Autodesk Fusion 360 part; units mm, degrees
sketch "Sketch1" plane through (0, 0, 0) normal (0, 0, 1) x (1, 0, 0)
  line L0 (10, 20.25) -> (-10, 20.25)
  line L1 (-10, 20.25) -> (-10, -20.25)
  line L2 (-10, -20.25) -> (10, -20.25)
  line L3 (10, -20.25) -> (10, 20.25)
  line L4 (10, 20.25) -> (-10, -20.25) construction
  line L5 (-10, 20.25) -> (10, -20.25) construction
  dimension "d1" = 20
  dimension "d2" = 40.5
extrude "Extrude1" add sketch "Sketch1" along normal blind 21.5
sketch "Sketch2" plane through (0, 0, 21.5) normal (0, 0, 1) x (-1, 0, 0)
  line L0 (-10, 20.25) -> (-10, -20.25)
  line L1 (-10, -20.25) -> (10, -20.25)
  line L2 (10, -20.25) -> (10, 20.25)
  line L3 (10, 20.25) -> (-10, 20.25)
  line L4 (-8, -18.25) -> (8, -18.25)
  line L5 (8, -18.25) -> (8, 18.25)
  line L6 (8, 18.25) -> (-8, 18.25)
  line L7 (-8, 18.25) -> (-8, -18.25)
  line L8 (-8, -18.25) -> (8, 18.25) construction
  line L9 (8, -18.25) -> (-8, 18.25) construction
  line L10 (-9, -19.25) -> (9, -19.25)
  line L11 (9, -19.25) -> (9, 19.25)
  line L12 (9, 19.25) -> (-9, 19.25)
  line L13 (-9, 19.25) -> (-9, -19.25)
  line L14 (-9, -19.25) -> (9, 19.25) construction
  line L15 (9, -19.25) -> (-9, 19.25) construction
  dimension "d5" = 1
  dimension "d6" = 1
  dimension "d7" = 1
  dimension "d8" = 1
extrude "Extrude2" add sketch "Sketch2" along normal blind 1 contours L10 L11 L12 L13
sketch "Sketch3" plane through (0, 0, 21.5) normal (0, 0, 1) x (-1, 0, 0)
  line L0 (-8, -18.25) -> (8, -18.25)
  line L1 (8, -18.25) -> (8, 18.25)
  line L2 (8, 18.25) -> (-8, 18.25)
  line L3 (-8, 18.25) -> (-8, -18.25)
  circle A0 centre (0, 10.25) radius 2
  line L4 (10, 20.25) -> (-10, 20.25)
  circle A1 centre (0, -0.75) radius 0.75
  circle A2 centre (0, -10.25) radius 3
  line L5 (-10, -20.25) -> (10, -20.25)
  circle A3 centre (0, -10.25) radius 4
  circle A4 centre (0, 10.25) radius 4
  dimension "d11" = 4
  dimension "d12" = 10
  dimension "d13" = 11
  dimension "d14" = 9.5
  dimension "d16" = 10
  dimension "d17" = 1.5
  dimension "d18" = 6
  dimension "d19" = 8
  dimension "d20" = 8
extrude "Extrude3" add sketch "Sketch3" along normal blind 5 contours A3
extrude "Extrude4" add sketch "Sketch3" along normal blind 5 contours A4
sketch "Sketch4" plane through (0, 0, 26.5) normal (0, 0, 1) x (-1, 0, 0)
  circle A0 centre (0, 10.25) radius 2
  circle A1 centre (0, 10.25) radius 4
  circle A2 centre (0, 10.25) radius 3
  dimension "d25" = 6
extrude "Extrude5" cut sketch "Sketch4" against normal blind 2.5 contours A1
extrude "Extrude6" cut sketch "Sketch3" against normal blind 1.5 contours A1
sketch "Sketch5" plane through (0, 0, 0) normal (0, 0, -1) x (1, 0, 0)
  line L0 (10, -20.25) -> (10, 20.25)
  line L1 (10, 20.25) -> (-10, 20.25)
  line L2 (-10, 20.25) -> (-10, -20.25)
  line L3 (-10, -20.25) -> (10, -20.25)
  line L4 (7.5, 18) -> (-7.5, 18) construction
  line L5 (-7.5, 18) -> (-7.5, -18) construction
  line L6 (-7.5, -18) -> (7.5, -18) construction
  line L7 (7.5, -18) -> (7.5, 18) construction
  line L8 (7.5, 18) -> (-7.5, -18) construction
  line L9 (-7.5, 18) -> (7.5, -18) construction
  circle A0 centre (-7.5, 18) radius 0.875
  circle A1 centre (7.5, 18) radius 0.875
  circle A2 centre (7.5, -18) radius 0.875
  circle A3 centre (-7.5, -18) radius 0.875
  dimension "d30" = 15
  dimension "d31" = 36
  dimension "d32" = 1.75
extrude "Extrude7" cut sketch "Sketch5" against normal blind 27 contours A0 | A1 | A2 | A3
sketch "Sketch6" plane through (0, 0, 0) normal (0, 0, -1) x (1, 0, 0)
  circle A0 centre (7.5, 18) radius 0.875
  circle A1 centre (7.5, -18) radius 0.875
  circle A2 centre (-7.5, 18) radius 0.875
  circle A3 centre (-7.5, -18) radius 0.875
  line L0 (10, -20.25) -> (10, 20.25)
  line L1 (10, 20.25) -> (-10, 20.25)
  line L2 (-10, 20.25) -> (-10, -20.25)
  line L3 (-10, -20.25) -> (10, -20.25)
  circle A4 centre (-7.5, 18) radius 1.875
  circle A5 centre (7.5, 18) radius 1.875
  circle A6 centre (7.5, -18) radius 1.875
  circle A7 centre (-7.5, -18) radius 1.875
  line L4 (9, 19.25) -> (-9, 19.25)
  line L5 (-9, 19.25) -> (-9, -19.25)
  line L6 (-9, -19.25) -> (9, -19.25)
  line L7 (9, -19.25) -> (9, 19.25)
  line L8 (9, 19.25) -> (-9, -19.25) construction
  line L9 (-9, 19.25) -> (9, -19.25) construction
  dimension "d35" = 3.75
  dimension "d36" = 1
  dimension "d37" = 1
extrude "Extrude8" cut sketch "Sketch6" against normal up to surface (19.5 mm away) contours A4 A5 A6 A7 L4 L5 L6 L7
extrude "Extrude9" cut 1 faces at (0.1483, -10.9, 21.5) along direction (0, 0, -1) blind 15
sketch "Sketch8" plane through (0, 0, 26.5) normal (0, 0, 1) x (-1, 0, 0)
  circle A0 centre (0, -10.25) radius 3
  circle A1 centre (0, -10.25) radius 4
  circle A2 centre (0, -10.25) radius 4
extrude "Extrude10" add sketch "Sketch8" against normal blind 2.5 contours A0
ref_plane "WorkPlane1" through (0, 6.25, 22) normal (0, -1, 0) x (1, 0, 0)
sketch "Sketch10" plane through (0, 6.25, 22) normal (0, -1, 0) x (1, 0, 0)
  line L0 (-4, 2) -> (4, 2)
  line L1 (4, 2) -> (4, -0.5)
  line L2 (4, -0.5) -> (-4, -0.5)
  line L3 (-4, -0.5) -> (-4, 2)
extrude "Extrude11" cut sketch "Sketch10" against normal blind 2
sketch "Sketch11" plane through (0, 0, 26.5) normal (0, 0, 1) x (-1, 0, 0)
  circle A0 centre (0, -10.25) radius 4
  circle A1 centre (0, -10.25) radius 0.75
  dimension "d47" = 1.5
extrude "Extrude12" cut sketch "Sketch11" against normal blind 1.5 contours A1
sketch "Sketch12" plane through (0, 0, 21.5) normal (0, 0, 1) x (-1, 0, 0)
  arc A0 (-3.4641, -8.25) -> (3.4641, -8.25) centre (0, -10.25) ccw
  line L0 (-3.4641, -8.25) -> (-2.2361, -8.25)
  arc A1 (-2.2361, -8.25) -> (2.2361, -8.25) centre (0, -10.25) ccw
  line L1 (2.2361, -8.25) -> (3.4641, -8.25)
  arc A2 (-8, 17.2819) -> (-6.6615, 18.25) centre (-7.5, 18) ccw
  line L2 (-8, 17.2819) -> (-8, -17.2819)
  arc A3 (-6.6615, -18.25) -> (-8, -17.2819) centre (-7.5, -18) ccw
  line L3 (-6.6615, -18.25) -> (6.6615, -18.25)
  arc A4 (8, -17.2819) -> (6.6615, -18.25) centre (7.5, -18) ccw
  line L4 (8, -17.2819) -> (8, 17.2819)
  arc A5 (6.6615, 18.25) -> (8, 17.2819) centre (7.5, 18) ccw
  line L5 (6.6615, 18.25) -> (-6.6615, 18.25)
  circle A6 centre (0, -0.75) radius 0.75
  circle A7 centre (0, 10.25) radius 4
  circle A8 centre (0, -10.25) radius 3
  dimension "d50" = 6
extrude "Extrude13" cut sketch "Sketch12" against normal blind 4 contours A1 A8
sketch "Sketch13" plane through (0, 0, 21.5) normal (0, 0, 1) x (-1, 0, 0)
  arc A0 (2.2361, -8.25) -> (-2.2361, -8.25) centre (0, -10.25) ccw
  line L0 (2.2361, -8.25) -> (3.4641, -8.25)
  arc A1 (-3.4641, -8.25) -> (3.4641, -8.25) centre (0, -10.25) ccw
  line L1 (-3.4641, -8.25) -> (-2.2361, -8.25)
  arc A2 (-8, 17.2819) -> (-6.6615, 18.25) centre (-7.5, 18) ccw
  line L2 (-8, 17.2819) -> (-8, -17.2819)
  arc A3 (-6.6615, -18.25) -> (-8, -17.2819) centre (-7.5, -18) ccw
  line L3 (-6.6615, -18.25) -> (6.6615, -18.25)
  arc A4 (8, -17.2819) -> (6.6615, -18.25) centre (7.5, -18) ccw
  line L4 (8, -17.2819) -> (8, 17.2819)
  arc A5 (6.6615, 18.25) -> (8, 17.2819) centre (7.5, 18) ccw
  line L5 (6.6615, 18.25) -> (-6.6615, 18.25)
  circle A6 centre (0, -0.75) radius 0.75
  circle A7 centre (0, 10.25) radius 4
  line L6 (-12.9231, -4.25) -> (12.9231, -4.25)
  line L7 (12.9231, -4.25) -> (12.9231, 2.75)
  line L8 (12.9231, 2.75) -> (-12.9231, 2.75)
  line L9 (-12.9231, 2.75) -> (-12.9231, -4.25)
  line L10 (-12.9231, -4.25) -> (12.9231, 2.75) construction
  line L11 (12.9231, -4.25) -> (-12.9231, 2.75) construction
  point P0 (0, -0.75)
  dimension "d53" = 7
extrude "Extrude14" cut sketch "Sketch13" along normal blind 3 contours L2 L6 L8 L9 | L4 L6 L7 L8
fillet "Fillet1" radius 0.35 8 edges at (-9, 4.25, 22) (-8, 4.25, 22) (-9, -2.75, 22) (-8, -2.75, 22) (8, 4.25, 22) (9, 4.25, 22) (8, -2.75, 22) (9, -2.75, 22)
fillet "Fillet2" radius 1 4 edges at (-10, -20.25, 10.75) (10, -20.25, 10.75) (-10, 20.25, 10.75) (10, 20.25, 10.75)
sketch "Sketch14" plane through (0, 0, 19.5) normal (0, 0, -1) x (1, 0, 0)
  circle A0 centre (0, -10.25) radius 3
  circle A1 centre (0, 10.25) radius 2
  arc A2 (-6.1025, -19.25) -> (-9, -16.875) centre (-7.5, -18) ccw
  line L0 (-6.1025, -19.25) -> (6.1025, -19.25)
  arc A3 (9, -16.875) -> (6.1025, -19.25) centre (7.5, -18) ccw
  line L1 (9, -16.875) -> (9, 16.875)
  arc A4 (6.1025, 19.25) -> (9, 16.875) centre (7.5, 18) ccw
  line L2 (6.1025, 19.25) -> (-6.1025, 19.25)
  arc A5 (-9, 16.875) -> (-6.1025, 19.25) centre (-7.5, 18) ccw
  line L3 (-9, 16.875) -> (-9, -16.875)
  circle A6 centre (0, -10.25) radius 8.5
  circle A7 centre (0, -10.25) radius 9.5
  dimension "d60" = 17
  dimension "d61" = 1
extrude "Extrude15" add sketch "Sketch14" along normal blind 12 contours A2 L0 A3 L1 L3 A7
sketch "Sketch15" plane through (0, 0, 19.5) normal (0, 0, -1) x (1, 0, 0)
  circle A0 centre (0, 10.25) radius 2
  arc A1 (9, -7.2086) -> (-9, -7.2086) centre (0, -10.25) ccw
  line L0 (9, -7.2086) -> (9, 16.875)
  arc A2 (6.1025, 19.25) -> (9, 16.875) centre (7.5, 18) ccw
  line L1 (6.1025, 19.25) -> (-6.1025, 19.25)
  arc A3 (-9, 16.875) -> (-6.1025, 19.25) centre (-7.5, 18) ccw
  line L2 (-9, 16.875) -> (-9, -7.2086)
  line L3 (5, 15.75) -> (-5, 15.75)
  line L4 (-5, 15.75) -> (-5, 4.75)
  line L5 (-5, 4.75) -> (5, 4.75)
  line L6 (5, 4.75) -> (5, 15.75)
  line L7 (5, 15.75) -> (-5, 4.75) construction
  line L8 (-5, 15.75) -> (5, 4.75) construction
  line L9 (6, 16.75) -> (-6, 16.75)
  line L10 (-6, 16.75) -> (-6, 3.75)
  line L11 (-6, 3.75) -> (6, 3.75)
  line L12 (6, 3.75) -> (6, 16.75)
  line L13 (6, 16.75) -> (-6, 3.75) construction
  line L14 (-6, 16.75) -> (6, 3.75) construction
  point P0 (0, 10.25)
  point P1 (0, 10.25)
  dimension "d64" = 10
  dimension "d65" = 11
  dimension "d66" = 1
  dimension "d67" = 1
extrude "Extrude16" add sketch "Sketch15" along normal blind 5 contours L9 L10 L11 L12
equation "d35 = 1.75 mm + 2 mm"
Input: part model. Units: mm. Frame: model coordinates. A direction names the side the tool comes from. Round coordinates to 2 decimals unless told otherwise and drop trailing zeros. Write each loop counter-clockwise with the first axis right and the second up, starting at its lowest first coordinate (ties: lowest second). Pieces come first, ordered by that corner, then holes. Notation, with made-up numbers: (63.25, 16.5) - (84.25, 16.5) arc R33 cw to (84.25, 48.5) - close; hole circle Ø6 at (18, 46). An arc over 180 degrees is marked (long way). Write item = value, one per line.
(1) Access query for faces 1 (the flat face through (5, 3, 7.5)), 2 (the flat face through (-9, 12, 22)), 3 (the flat face through (9, -11, 22)), 4 (the flat face through (3, -12, 24)). Directions: +Z, -Z, +X, -X, +Y, -Y. A direction counts if a zero-diameter tool reaches every point of the face in a straight line with its end or side. Return the directions, or none.
Geometry check:
face_1 = -Z
face_2 = +Z, -X, +Y, -Y
face_3 = +Z, +X, +Y, -Y
face_4 = +Z
(2) Section query A-A on z = 23. Output: boundary loops of the cut face in (x, y), then the cut area to 3 significant figures.
Geometry check:
outline = circle Ø8 at (0, -10.25); (-3.46, 8.25) - (-2.24, 8.25) arc R3 cw (long way) to (2.24, 8.25) - (3.46, 8.25) arc R4 ccw (long way) to start; hole circle Ø4 at (0, -10.25)
area = 53.0 mm^2
(3) Material intervals for probe 1 along Y at (x, z) = (-7.5, 6) (3 decimals); probe 2 along X at (y, z) = (-12.5, 17.5); probe 3 along Y at (x, z) = (0, 14.25), sorted ascending.
Geometry check:
probe_1 = -20.25 to -18.875, -17.125 to -16.125, 16.125 to 17.125, 18.875 to 20.25
probe_2 = -10 to -9, -6 to -5, 5 to 6, 9 to 10
probe_3 = -20.25 to -19.25, 0.75 to 1.75, 18.75 to 20.25
(4) Section query C-C on z = 4. Output: boundary loops of the cut face in (x, y) (3 decimals), then the cut area to 3 significant figures.
Geometry check:
outline = (-10, -19.25) arc R1 ccw to (-9, -20.25) - (9, -20.25) arc R1 ccw to (10, -19.25) - (10, 19.25) arc R1 ccw to (9, 20.25) - (-9, 20.25) arc R1 ccw to (-10, 19.25) - close; hole (-9, -16.875) arc R1.875 cw (long way) to (-6.102, -19.25) - (6.102, -19.25) arc R1.875 cw (long way) to (9, -16.875) - (9, 16.875) arc R1.875 cw (long way) to (6.102, 19.25) - (-6.102, 19.25) arc R1.875 cw (long way) to (-9, 16.875) - close; hole circle Ø1.75 at (-7.5, -18); hole circle Ø1.75 at (-7.5, 18); hole circle Ø1.75 at (7.5, -18); hole circle Ø1.75 at (7.5, 18)
area = 144 mm^2
(5) Contact query for flat-ended pins moving along their axis: pin 1 Ø1.1 at (x, y) = (7.5, 18) entering from +Z; pin 2 Ø3 at (x, y) = (-3, 4) entering from -Z; pin 3 Ø1.5 at (x, y) = (-2, 0.5) entering from +Z; pin 4 Ø1.4 at (x, z) = (-2.5, 22.5) entering from -Y. Output: stop coordinate, or through.
Geometry check:
pin_1 = through
pin_2 = 19.5
pin_3 = 21.5
pin_4 = -19.25
(6) Pull-direction query (X, two-part tool) for faces 5 (the flat face through (0, -3.75, 17)), 6 (the cylindrical face through (9.699, -19.965, 10.901)), 7 (the cylindrical face through (2.997, -10.382, 25.268)); classes: +X half, -X half, draft (parallel to the pull), parting line (faces both ways), or undercut.
Geometry check:
face_5 = undercut
face_6 = +X half
face_7 = parting line
(7) Section query D-D on x = 0. State how many separate pieces and enclosed holes the cut face has, then the cut area to 3 significant figures.
Geometry check:
separate_pieces = 3
enclosed_holes = 0
area = 163 mm^2
